Check sheet for the drawn part. Datum: minimum x, y, z corner. Units: mm. A direction names the side the tool comes from. Round coordinates to 2 decimals unless told otherwise and drop trailing zeros. Order: outer loops, then holes, each group sorted by start corner. A loop starts at its lowest first (then second) coordinate and runs counter-clockwise, first axis right, second up. Notation, with made-up numbers: (42.25, -21.75) -> (88.25, -21.75) arc R27 ccw to (88.25, 5.25) -> close; hole circle Ø1 at (21.5, 19). An arc over 180 degrees is marked (long way). Write item = value, one per line. Start each with the question number.
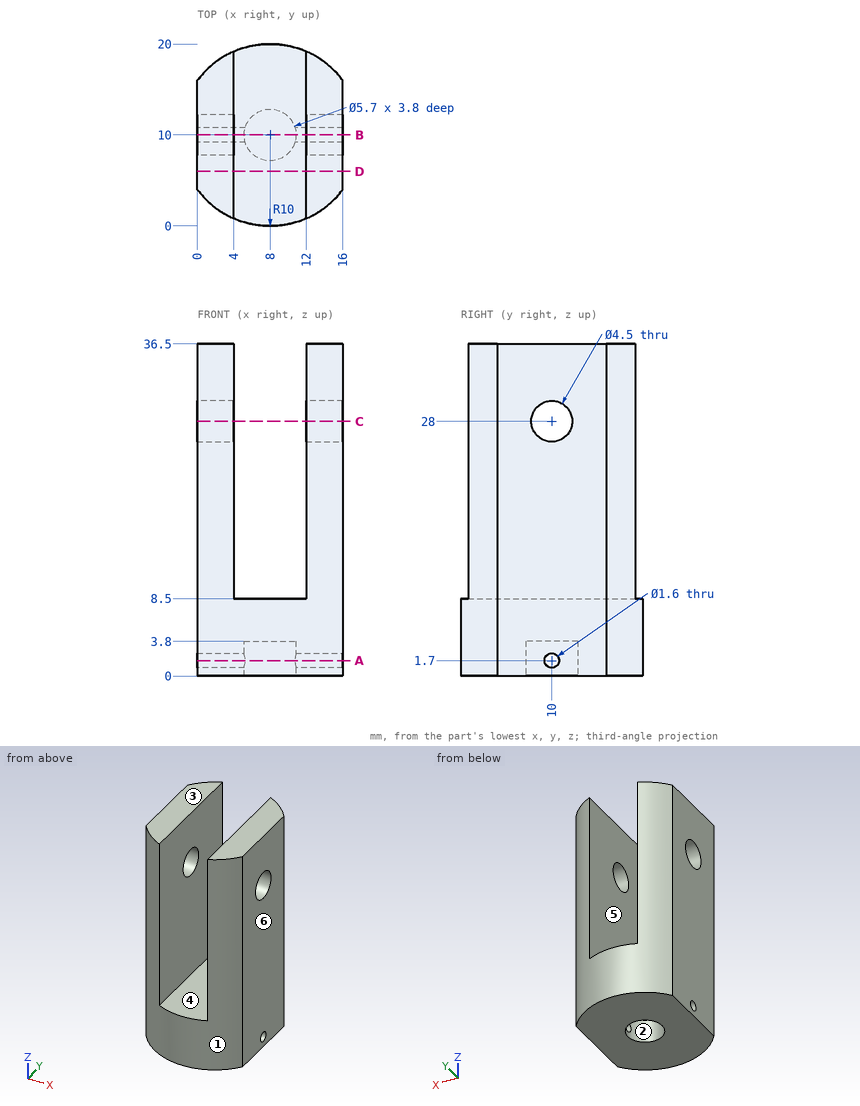
(1) Scan lines: line 1 along Z through (x, y) = (2.9, 10); line 2 along X through (y, z) = (12.25, 33); line 3 along Z through (x, y) = (6.25, 16). Record each from-to range of solid material in increasing order. Write a range as from..to.
(2) Depth check by flat-ended pin: pin 1 (3.5 mm diameter, centred on x = 8, y = 10, fed in from -Z); pin 2 (6 mm diameter, centred on x = 12.5, z = 11.5, fed in from +Y); pin 3 (6 mm diameter, centred on x = 4.5, y = 12.5, fed in from +Z); pin 4 (6 mm diameter, centred on x = 7.5, y = 6.5, fed in from +Z). Enter the tip coordinate at first touch or a pass-through.
(3) Draft check along X on the marked faces 1, 2, 3 and 4. Enter one of: +X half, -X half, draft (parallel to the pull), parting line (faces both ways), or undercut.
(4) Cross-section at A-A (z = 1.7). Enter the section's corners in (x, y), and give its area (3 significant figures).
(5) Cross-section at B-B (y = 10). Enter the section's corners in (x, z), and give its area (3 significant figures).
(6) Cross-section at C-C (z = 28). Enter the section's corners in (x, y).
(7) Cross-section at D-D (y = 6). Enter the section's corners in (x, z), and give its area (3 significant figures).
(8) Set-up check for the marked faces 5 and 6: record each of +Z, -Z, +X, -X, +Y, -Y from which the full face is reachable in a straight line by a thin tool's end or side.
Outcome:
q1.line_1 = 0..0.9, 2.5..25.75, 30.25..36.5
q1.line_2 = 0..4, 12..16
q1.line_3 = 0..8.5
q2.pin_1 = 3.8
q2.pin_2 = 19.17
q2.pin_3 = 36.5
q2.pin_4 = 8.5
q3.face_1 = parting line
q3.face_2 = undercut
q3.face_3 = draft
q3.face_4 = undercut
q4.outline = (0, 4) arc R10 ccw to (16, 4) -> (16, 9.2) -> (10.74, 9.2) arc R2.85 cw to (5.26, 9.2) -> (0, 9.2) -> close; (0, 10.8) -> (5.26, 10.8) arc R2.85 cw to (10.74, 10.8) -> (16, 10.8) -> (16, 16) arc R10 ccw to (0, 16) -> close
q4.area = 239 mm^2
q5.outline = (0, 0) -> (5.15, 0) -> (5.15, 0.9) -> (0, 0.9) -> close; (0, 2.5) -> (5.15, 2.5) -> (5.15, 3.8) -> (10.85, 3.8) -> (10.85, 2.5) -> (16, 2.5) -> (16, 25.75) -> (12, 25.75) -> (12, 8.5) -> (4, 8.5) -> (4, 25.75) -> (0, 25.75) -> close; (0, 30.25) -> (4, 30.25) -> (4, 36.5) -> (0, 36.5) -> close; (10.85, 0) -> (16, 0) -> (16, 0.9) -> (10.85, 0.9) -> close; (12, 30.25) -> (16, 30.25) -> (16, 36.5) -> (12, 36.5) -> close
q5.area = 286 mm^2
q6.outline = (0, 4) arc R10 ccw to (4, 0.83) -> (4, 7.75) -> (0, 7.75) -> close; (0, 12.25) -> (4, 12.25) -> (4, 19.17) arc R10 ccw to (0, 16) -> close; (12, 0.83) arc R10 ccw to (16, 4) -> (16, 7.75) -> (12, 7.75) -> close; (12, 12.25) -> (16, 12.25) -> (16, 16) arc R10 ccw to (12, 19.17) -> close
q7.outline = (0, 0) -> (16, 0) -> (16, 36.5) -> (12, 36.5) -> (12, 8.5) -> (4, 8.5) -> (4, 36.5) -> (0, 36.5) -> close
q7.area = 360 mm^2
q8.face_5 = +Z, +Y, -Y
q8.face_6 = +Z, -Z, +X, +Y, -Y
